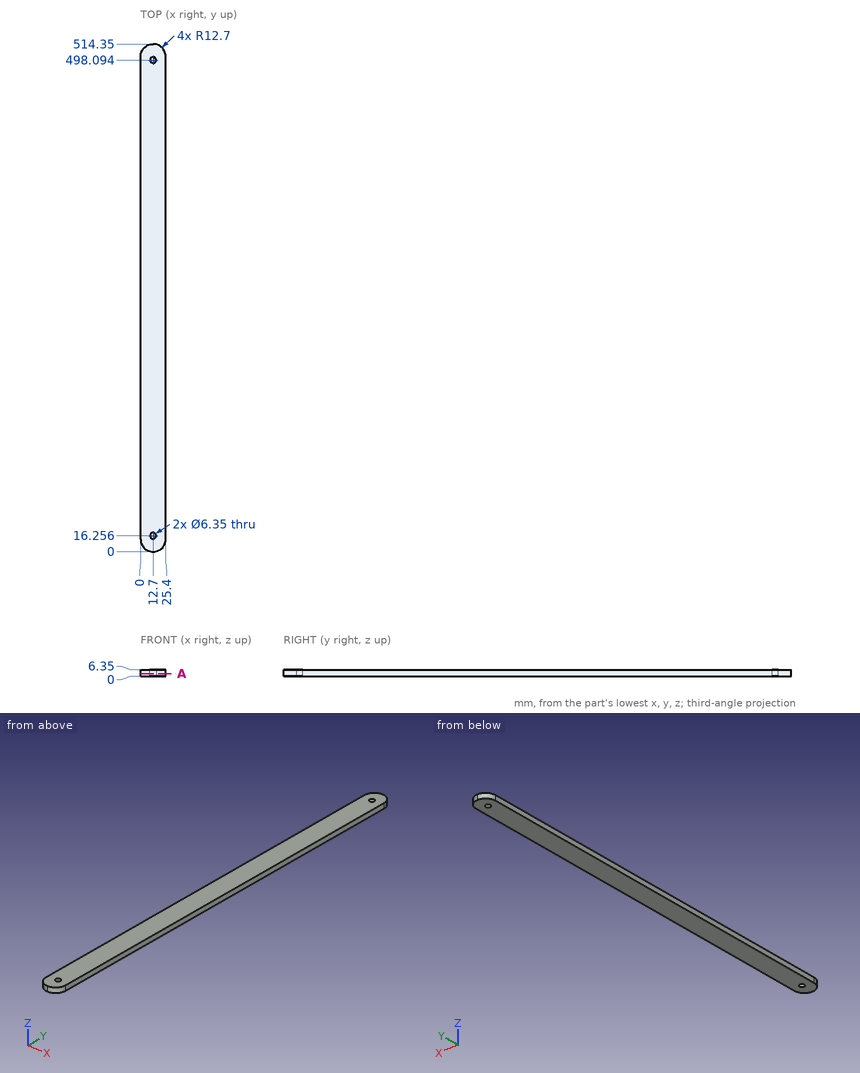
The figure shows three views and two pictorial views of one solid part (mm, origin at its lowest corner). Answer the questions. Coordinates: 2 decimals unless noted, no trailing zeros. Use CSV: the item, a comma, the result in double quotes. Start each with the question number.
(1) Find section A-A, the plane z = 2.5. State how many separate pieces and enclosed holes the cut face has, then the cut area to 3 significant figures.
(2) Consider line 1 (Y direction, x = 13.25, z = 3.25); line 2 (Y direction, x = 12.7, z = 2); line 3 (Y direction, x = 23.25, z = 6). Determine where each line is inside the solid, lowest interval first.
(3) Given pin 1 Ø1 at (x, z) = (4.5, 5.5) entering from -Y, flat-ended and moving along its own axis, determine where the tip first touches the part or whether it passes through.
Recorded:
1,separate pieces,"1"
1,enclosed holes,"2"
1,area,"12,900 mm^2"
2,line 1,"y = 0.01 to 13.13, 19.38 to 494.97, 501.22 to 514.34"
2,line 2,"y = 0 to 13.08, 19.43 to 494.92, 501.27 to 514.35"
2,line 3,"y = 5.63 to 508.72"
3,pin 1,"stops at y = 2.6"
